```python
from build123d import *

# Parameters (mm, degrees)
F0_R           = 11
F1_DEPTH       = 3
F2_D           = 5.85
F2_CBORE_D     = 10
F2_CBORE_DEPTH = 1.8
F3_D           = 5
F3_CBORE_D     = 10
F3_CBORE_DEPTH = 2


# Not quite as in the source:
# - a feature names something its author has since deleted; it is built from what else it names


with BuildPart() as f1:
    # F0 (on Top) → F1 (new body)
    with BuildSketch(Plane.XY):
        with BuildLine():
            Line((18.85, 13.75), (-18.85, 13.75))
            ThreePointArc((-18.85, 13.75), (-32.6, 0), (-18.85, -13.75))
            Line((-18.85, -13.75), (18.85, -13.75))
            ThreePointArc((18.85, -13.75), (32.6, 0), (18.85, 13.75))
        make_face()
        Circle(F0_R, mode=Mode.SUBTRACT)
    extrude(amount=-F1_DEPTH)

    # F2 (through all)
    with Locations(Plane.XY):
        with Locations((24.1, 0), (-24.1, 0)):
            CounterBoreHole(F2_D / 2, F2_CBORE_D / 2, F2_CBORE_DEPTH)

    # F3 (through all)
    with Locations(Plane.XY):
        with Locations((-15.6095083693, 7.4526413832), (-15.6095083693, -7.4526413832), (15.6095083693, -7.4526413832), (15.6095083693, 7.4526413832)):
            CounterBoreHole(F3_D / 2, F3_CBORE_D / 2, F3_CBORE_DEPTH)


solid = f1.part
```
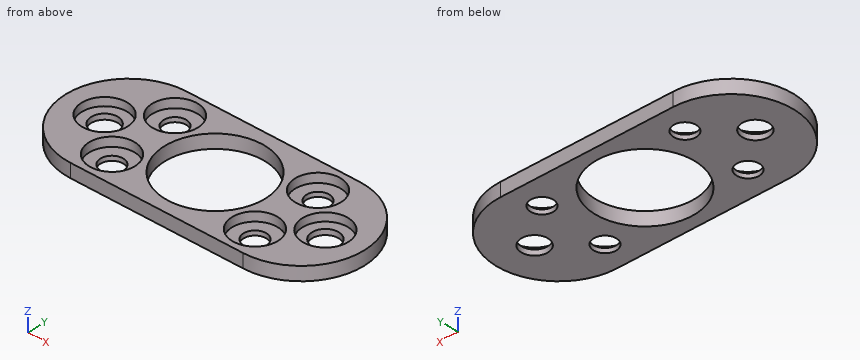
Source: CAD feature listing. Evaluate the final solid. Frame: model axes, mm. Give positions to 0.01 mm unless a question says otherwise; leave off trailing zeros. Loops run counter-clockwise (first coordinate to the right, second up) from the corner with the lowest first, then second, coordinate; pieces in that order, holes last. Notation, with made-up numbers: (67.25, -13) -> (99.25, -13) arc R23 cw to (99.25, 13) -> close; hole circle Ø3 at (58, 82.5). An arc over 180 degrees is marked (long way). Put each result on its own line as item: value. Start each with the question number.
1) Contact query for flat-ended pins moving along their axis: P1, Ø4, axis at x = 15.61, y = -7.45, coming from the -Z side; P2, Ø3, axis at x = 17, y = 7.5, coming from the +Z side; P3, Ø3, axis at x = 24, y = -2.5, coming from the +Z side. Output: stop coordinate, or through.
2) Cut plane D-D (y = -8.75). Return loops of the section in (x, z), then the cut area to 3 significant figures.
3) Cut plane C-C (z = -1.35). Return loops of the section in (x, y).
4) Material intervals for probe 1 along Y at (x, z) = (-0.5, -0.4); probe 2 along X at (y, z) = (-8, -2.65); probe 3 along X at (y, z) = (-8.5, -0.75), sorted ascending.
5) Cut plane A-A (x = 0). Return loops of the section in (y, z), then the cut area to 3 significant figures.
6) Cut plane B-B (y = 0). Return loops of the section in (x, z) (3 decimals), then the cut area to 3 significant figures.
Results are:
1. P1: passes through
1. P2: stops at z = -2
1. P3: stops at z = -1.8
2. outline: (-29.46, -3) -> (-17.75, -3) -> (-17.75, -2) -> (-20.44, -2) -> (-20.44, 0) -> (-29.46, 0) -> close; (-13.47, -3) -> (-6.67, -3) -> (-6.67, 0) -> (-10.78, 0) -> (-10.78, -2) -> (-13.47, -2) -> close; (6.67, -3) -> (13.47, -3) -> (13.47, -2) -> (10.78, -2) -> (10.78, 0) -> (6.67, 0) -> close; (17.75, -3) -> (29.46, -3) -> (29.46, 0) -> (20.44, 0) -> (20.44, -2) -> (17.75, -2) -> close
2. area: 89.6 mm2
3. outline: (-18.85, -13.75) -> (18.85, -13.75) arc R13.75 ccw to (18.85, 13.75) -> (-18.85, 13.75) arc R13.75 ccw to start; hole circle Ø10 at (-24.1, 0); hole circle Ø10 at (-15.61, -7.45); hole circle Ø10 at (-15.61, 7.45); hole circle Ø22 at (0, 0); hole circle Ø10 at (15.61, -7.45); hole circle Ø10 at (15.61, 7.45); hole circle Ø10 at (24.1, 0)
4. probe 1: y = -13.75 to -10.99, 10.99 to 13.75
4. probe 2: x = -30.03 to -18.05, -13.17 to -7.55, 7.55 to 13.17, 18.05 to 30.03
4. probe 3: x = -29.66 to -20.5, -10.72 to -6.98, 6.98 to 10.72, 20.5 to 29.66
5. outline: (-13.75, -3) -> (-11, -3) -> (-11, 0) -> (-13.75, 0) -> close; (11, -3) -> (13.75, -3) -> (13.75, 0) -> (11, 0) -> close
5. area: 16.5 mm2
6. outline: (-32.6, -3) -> (-27.025, -3) -> (-27.025, -1.8) -> (-29.1, -1.8) -> (-29.1, 0) -> (-32.6, 0) -> close; (-21.175, -3) -> (-11, -3) -> (-11, 0) -> (-19.1, 0) -> (-19.1, -1.8) -> (-21.175, -1.8) -> close; (11, -3) -> (21.175, -3) -> (21.175, -1.8) -> (19.1, -1.8) -> (19.1, 0) -> (11, 0) -> close; (27.025, -3) -> (32.6, -3) -> (32.6, 0) -> (29.1, 0) -> (29.1, -1.8) -> (27.025, -1.8) -> close
6. area: 79.6 mm2
